from build123d import *

# Parameters (mm, degrees)
F0_W     = 25.4
F0_H     = 19.05
F1_DEPTH = 3.175


# Not quite as in the source:
# - a feature names something its author has since deleted; it is built from what else it names


with BuildPart() as f1:
    # F0 (on Top) → F1 (new body)
    with BuildSketch(Plane.XY):
        Polygon((2.0699514867, -0.1923768919), (2.0699514867, 50.6076231081), (-61.4300485133, 50.6076231081), (-64.6050485133, 50.6076231081), (-64.6050485133, 25.2076231081), (-61.4300485133, 25.2076231081), (-61.4300485133, 13.9046231081), (-58.8900485133, 13.9046231081), (-58.8900485133, 15.9366231081), (-56.3500485133, 15.9366231081), (-56.3500485133, 13.9046231081), (-53.8100485133, 13.9046231081), (-53.8100485133, 11.1106231081), (-56.3500485133, 11.1106231081), (-56.3500485133, 9.0786231081), (-58.8900485133, 9.0786231081), (-58.8900485133, 11.1106231081), (-61.4300485133, 11.1106231081), (-61.4300485133, -0.1923768919), (-64.6050485133, -0.1923768919), (-64.6050485133, -25.5923768919), (-61.4300485133, -25.5923768919), (-61.4300485133, -36.8953768919), (-58.8900485133, -36.8953768919), (-58.8900485133, -34.8633768919), (-56.3500485133, -34.8633768919), (-56.3500485133, -36.8953768919), (-53.8100485133, -36.8953768919), (-53.8100485133, -39.6893768919), (-56.3500485133, -39.6893768919), (-56.3500485133, -41.7213768919), (-58.8900485133, -41.7213768919), (-58.8900485133, -39.6893768919), (-61.4300485133, -39.6893768919), (-61.4300485133, -50.9923768919), (-36.0300485133, -50.9923768919), (-36.0300485133, -35.7523768919), (-20.7900485133, -35.7523768919), (-20.7900485133, -47.8173768919), (-9.4870485133, -47.8173768919), (-9.4870485133, -45.2773768919), (-11.5190485133, -45.2773768919), (-11.5190485133, -42.7373768919), (-9.4870485133, -42.7373768919), (-9.4870485133, -40.1973768919), (-6.6930485133, -40.1973768919), (-6.6930485133, -42.7373768919), (-4.6610485133, -42.7373768919), (-4.6610485133, -45.2773768919), (-6.6930485133, -45.2773768919), (-6.6930485133, -47.8173768919), (4.6099514867, -47.8173768919), (4.6099514867, -50.9923768919), (30.0099514867, -50.9923768919), (30.0099514867, -47.8173768919), (41.3129514867, -47.8173768919), (41.3129514867, -45.2773768919), (39.2809514867, -45.2773768919), (39.2809514867, -42.7373768919), (41.3129514867, -42.7373768919), (41.3129514867, -40.1973768919), (44.1069514867, -40.1973768919), (44.1069514867, -42.7373768919), (46.1389514867, -42.7373768919), (46.1389514867, -45.2773768919), (44.1069514867, -45.2773768919), (44.1069514867, -47.8173768919), (55.4099514867, -47.8173768919), (55.4099514867, -50.9923768919), (80.8099514867, -50.9923768919), (80.8099514867, -0.1923768919), align=None)
        with Locations((-31.2025573432, 25.8426231081)):
            Rectangle(F0_W, F0_H, mode=Mode.SUBTRACT)
    extrude(amount=F1_DEPTH)


solid = f1.part
Verification items for the finished model (mm, model axes). A direction names the side the tool comes from. Coordinates: 2 decimals unless noted, no trailing zeros. Order: outer loops, then holes, each group sorted by start corner. A loop starts at its lowest first (then second) coordinate and runs counter-clockwise, first axis right, second up.
1. Go/stop test with flat-tipped pins: pin 1 Ø1.5 at (y, z) = (-26.5, 1) entering from -X; pin 2 Ø1.6 at (x, z) = (34.5, 1.5) entering from -Y; pin 3 Ø0.8 at (y, z) = (12, 2) entering from -X. Record where each tip stops, or that it passes through.
Results found:
pin 1: stops at x = -61.43
pin 2: stops at y = -47.82
pin 3: stops at x = -53.81
2. Set-up check for faces 1 (the face through (-53.81, -38, 2)), 2 (the face through (-31, 35.368, 2)), 3 (the face through (-63, -25.592, 2)), 4 (the face through (4.61, -49, 2)), 5 (the face through (-9, -11, 3.175)): record each of +Z, -Z, +X, -X, +Y, -Y from which the full face is reachable in a straight line by a thin tool's end or side.
Results found:
face 1: +Z, -Z, -X
face 2: +Z, -Z
face 3: +Z, -Z, -X, -Y
face 4: +Z, -Z, -Y
face 5: +Z, +X, -X, +Y, -Y
3. Sectioned sample at B-B, the plane x = 20. Record the cut outline in (y, z) (3 decimals), and give its area (3 significant figures).
Results found:
outline: (-50.992, 0) - (-0.192, 0) - (-0.192, 3.175) - (-50.992, 3.175) - close
area: 161 mm2
4. Release check for a two-part mould opening along X. For faces 6 (the face through (-8, -40.197, 2)), 7 (the face through (-9, -11, 0)), 8 (the face through (-53.81, 13, 2)) record: +X half, -X half, draft (parallel to the pull), parting line (faces both ways), or undercut.
Results found:
face 6: undercut
face 7: draft
face 8: -X half
5. Scan lines: line 1 (X direction, y = -46.5, z = 0.3); line 2 (X direction, y = -41, z = 0.5); line 3 (X direction, y = -43.5, z = 0.6). Record each from-to range of solid material in increasing order.
Results found:
line 1: x = -61.43 to -36.03, -20.79 to -9.49, -6.69 to 41.31, 44.11 to 80.81
line 2: x = -61.43 to -58.89, -56.35 to -36.03, -20.79 to -9.49, -6.69 to 41.31, 44.11 to 80.81
line 3: x = -61.43 to -36.03, -20.79 to -11.52, -4.66 to 39.28, 46.14 to 80.81
6. Sectioned sample at A-A, the plane y = -30. Record the cut outline in (x, z) (3 decimals), and give its area (3 significant figures).
Results found:
outline: (-61.43, 0) - (80.81, 0) - (80.81, 3.175) - (-61.43, 3.175) - close
area: 452 mm2
